CAD build for the part. Positions are in the model's coordinates, mm. A direction names the side the tool comes from. Give positions to 0.01 mm unless a question says otherwise; leave off trailing zeros. Loops run counter-clockwise (first coordinate to the right, second up) from the corner with the lowest first, then second, coordinate; pieces in that order, holes last. Notation, with made-up numbers: M 49,23.5 L 68,23.5 A15 ccw 68,33.5 Z; hole C 22,69 d1. An arc over 180 degrees is marked long. One line per question, with ' | ' between items.
```python
from build123d import *

# Parameters (mm, degrees)
SKETCH_1_R      = 5.85
SKETCH_1_R_2    = 3.25
EXTRUDE_1_DEPTH = 22
CHAMFER_1_SIZE  = 1.5
EXTRUDE_START   = -10
EXTRUDE_2_DEPTH = 3
EXTRUDE_START_2 = 5
EXTRUDE_3_DEPTH = 3


with BuildPart() as part:
    # 草图1 → 凸台-拉伸1 (new body)
    with BuildSketch(Plane.XY):
        Circle(SKETCH_1_R)
        Circle(SKETCH_1_R_2, mode=Mode.SUBTRACT)
    extrude(amount=EXTRUDE_1_DEPTH)

    # 倒角1
    chamfer_1_edges = [part.edges().sort_by_distance(p)[0] for p in [
        (-5.85, 0, 22),
    ]]
    chamfer(chamfer_1_edges, length=CHAMFER_1_SIZE)

    # 草图2 → 凸台-拉伸2 (add)
    with BuildSketch(Plane.XY.offset(22).offset(EXTRUDE_START)):
        with BuildLine():
            Line((-3.173831975, 4.914192771), (-3.445099666, 5.334209247))
            ThreePointArc((-3.445099666, 5.334209247), (-6.246549311, -1.141543565), (-1.335802196, -6.207908866))
            Line((-1.335802196, -6.207908866), (-1.23062092, -5.719097145))
            ThreePointArc((-1.23062092, -5.719097145), (-5.754695034, -1.051658245), (-3.173831975, 4.914192771))
        make_face()
    extrude(amount=EXTRUDE_2_DEPTH)

    # 草图3 → 凸台-拉伸3 (add)
    with BuildSketch(Plane(origin=(0, 0, 12), x_dir=(-1, 0, 0), z_dir=(0, 0, -1)).offset(EXTRUDE_START_2)):
        with BuildLine():
            Line((1.23062092, -5.719097145), (1.335802196, -6.207908866))
            ThreePointArc((1.335802196, -6.207908866), (6.246549311, -1.141543565), (3.445099666, 5.334209247))
            Line((3.445099666, 5.334209247), (3.173831975, 4.914192771))
            ThreePointArc((3.173831975, 4.914192771), (5.754695034, -1.051658245), (1.23062092, -5.719097145))
        make_face()
    extrude(amount=-EXTRUDE_3_DEPTH)


solid = part.part
```
Item 1: Saw through at A-A on x = 0. Give the cut face in (y, z).
Conclusion:
outline: M -5.85,0 L -3.25,0 L -3.25,22 L -4.35,22 L -5.85,20.5 Z; M 3.25,0 L 5.85,0 L 5.85,20.5 L 4.35,22 L 3.25,22 Z
Item 2: Mould opens along Z. For faces 1 (the cylindrical face through (-6.265, -1.038, 13.479)), 2 (the flat face through (-6, -1, 7)), 3 (the flat face through (-6, -1, 15)), 4 (the flat face through (-6, -1, 10)) say: pulls with the +Z half, pulls with the -Z half, needs draft (parallel to the pull), parting line crosses it, or undercut.
Conclusion:
face 1: needs draft | face 2: pulls with the -Z half | face 3: pulls with the +Z half | face 4: undercut
Item 3: Drop flat-ended pins along their axis: P1, Ø3, axis at y = 2, z = 12, coming from the -X side; P2, Ø2, axis at y = -2.5, z = 14.5, coming from the -X side; P3, Ø6, axis at x = 3, z = 19.5, coming from the -Y side. Give the stop position or say it passes through.
Conclusion:
P1: x = -6.33 | P2: x = -6.17 | P3: y = -5.85
Item 4: 3-axis set-ups, long thin cutter, end or side, ignore diameter. For faces 5 (the flat face through (-6, -1, 12)), 6 (the cylindrical face through (5.58, 1.76, 10.11)), 7 (the flat face through (3, -3, 0)): which of +Z, -Z, +X, -X, +Y, -Y reach the whole face in a straight line?
Conclusion:
face 5: -X | face 6: none | face 7: -Z, +X, -X, +Y, -Y
Item 5: Saw through at C-C on z = 20.75. Give the cut face in (x, y).
Conclusion:
outline: C 0,0 d11.2; hole C 0,0 d6.5
Item 6: Drill centre lines: line 1 along Y through (x, z) = (0, 14.5); line 2 along X through (y, z) = (0.25, 19.25); line 3 along Z through (x, y) = (-4.25, 4.5). Where is each one in solid material? Low to high. Write a range as [from, to].
Conclusion:
line 1: [-5.85, -3.25], [3.25, 5.85] | line 2: [-5.84, -3.24], [3.24, 5.84] | line 3: [7, 10], [12, 15]
Item 7: Saw through at B-B on z = 8. Give the cut face in (x, y), and give its area (3 significant figures).
Conclusion:
outline: M -3.45,5.33 A6.35 ccw -1.34,-6.21 L -1.23,-5.72 A5.85 ccw long -3.17,4.91 Z; hole C 0,0 d6.5 | area: 81.5 mm²
